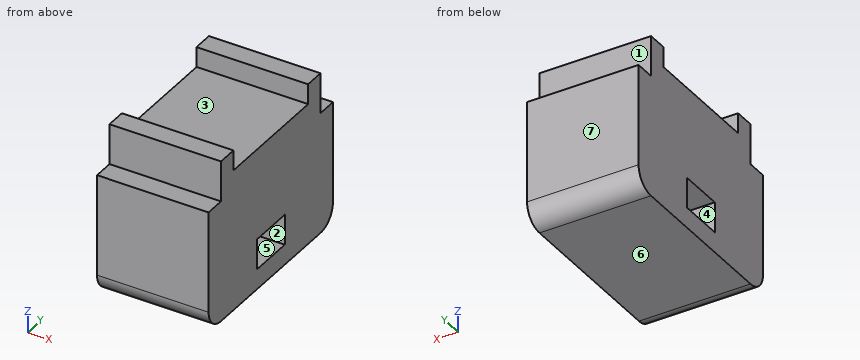
```python
from build123d import *

# Parameters (mm, degrees)
SKETCH1_W           = 20
SKETCH1_H           = 12
BOSS_EXTRUDE1_DEPTH = 11
SKETCH5_W           = 16
SKETCH5_H           = 11
BOSS_EXTRUDE2_DEPTH = 8
FILLET1_R           = 2
SKETCH7_W           = 4.5
SKETCH7_H           = 3
CUT_EXTRUDE1_DEPTH  = 15
SKETCH9_W           = 11
SKETCH9_H           = 2
BOSS_EXTRUDE4_DEPTH = 2


with BuildPart() as part:
    # Sketch1 → Boss-Extrude1 (new body)
    with BuildSketch(Plane.YZ):
        Rectangle(SKETCH1_W, SKETCH1_H)
    extrude(amount=BOSS_EXTRUDE1_DEPTH)

    # Sketch5 → Boss-Extrude2 (add)
    with BuildSketch(Plane(origin=(0, 0, 0), x_dir=(0, 1, 0), z_dir=(0, 0, 1))):
        with Locations((0, -5.5)):
            Rectangle(SKETCH5_W, SKETCH5_H)
    extrude(amount=BOSS_EXTRUDE2_DEPTH)

    # Fillet1
    fillet1_edges = [part.edges().sort_by_distance(p)[0] for p in [
        (5.5, 10, -6),
        (5.5, -10, -6),
    ]]
    fillet(fillet1_edges, radius=FILLET1_R)

    # Sketch7 → Cut-Extrude1 (cut)
    with BuildSketch(Plane.YZ):
        with Locations((0, -2.5)):
            Rectangle(SKETCH7_W, SKETCH7_H)
    extrude(amount=CUT_EXTRUDE1_DEPTH, mode=Mode.SUBTRACT)

    # Sketch9 → Boss-Extrude4 (add)
    with BuildSketch(Plane.XY.offset(8)):
        with Locations((5.5, 7)):
            Rectangle(SKETCH9_W, SKETCH9_H)
        with Locations((5.5, -7)):
            Rectangle(SKETCH9_W, SKETCH9_H)
    extrude(amount=BOSS_EXTRUDE4_DEPTH)


solid = part.part
```
CAD build for the part. Positions are in the model's coordinates, mm. Face numbers are marked on the shaded views. A direction names the side the tool comes from. Round coordinates to 2 decimals unless told otherwise and drop trailing zeros. Order: outer loops, then holes, each group sorted by start corner. A loop starts at its lowest first (then second) coordinate and runs counter-clockwise, first axis right, second up. Notation, with made-up numbers: (46, 30.5) - (51, 30.5) arc R14 ccw to (51, 38.5) - close; hole circle Ø10 at (43, 58.5). An arc over 180 degrees is marked (long way). Use CSV: the item, a comma, the result in double quotes. Start each with the question number.
1) Two-plate mould, pull along Z, no slides. Class the marked faces 4, 5, 6 and 7: pulls with the +Z half, pulls with the -Z half, needs draft (parallel to the pull), parting line crosses it, or undercut.
2) Saw through at B-B (y = 1). List the corners of the cut face in (x, z), and give its area (3 significant figures).
3) Saw through at D-D (y = 5.25). List the corners of the cut face in (x, z), and give its area (3 significant figures).
4) Saw through at A-A (z = -3.5). List the corners of the cut face in (x, y), and give its area (4 significant figures).
5) Pin check, flat tips, straight feed: pin 1 Ø1 at (y, z) = (7, 6.5) entering from -X; pin 2 Ø3.5 at (x, y) = (6.5, 0.5) entering from +Z; pin 3 Ø2 at (x, z) = (3, 8.5) entering from -Y; pin 4 Ø1.6 at (x, y) = (6.5, 9) entering from +Z. Stop position of each tip, or through.
6) Tool access for the marked faces 1, 2 and 3: list every direction of +Z, -Z, +X, -X, +Y, -Y with a clear straight run to the whole face (end or side of a thin tool).
7) Saw through at C-C (x = 4.25). List the corners of the cut face in (y, z).
8) Wall check: L1, parallel to Z at x = 4, y = 1.5; L2, parallel to Y at x = 5, z = -2; L3, parallel to Y at x = 8.25, z = 8.25. Give the ranges that are in metal, low to high. Write a range as [from, to].
Values follow:
1,face 4,"undercut"
1,face 5,"undercut"
1,face 6,"pulls with the -Z half"
1,face 7,"needs draft"
2,outline,"(0, -6) - (11, -6) - (11, -4) - (0, -4) - close; (0, -1) - (11, -1) - (11, 8) - (0, 8) - close"
2,area,"121 mm2"
3,outline,"(0, -6) - (11, -6) - (11, 8) - (0, 8) - close"
3,area,"154 mm2"
4,outline,"(0, -10) - (11, -10) - (11, -2.25) - (0, -2.25) - close; (0, 2.25) - (11, 2.25) - (11, 10) - (0, 10) - close"
4,area,"170.5 mm2"
5,pin 1,"stops at x = 0"
5,pin 2,"stops at z = 8"
5,pin 3,"stops at y = -8"
5,pin 4,"stops at z = 6"
6,face 1,"+Z, +X, -X, +Y"
6,face 2,"+X, -X"
6,face 3,"+Z, +X, -X"
7,outline,"(-10, -4) arc R2 ccw to (-8, -6) - (8, -6) arc R2 ccw to (10, -4) - (10, 6) - (8, 6) - (8, 10) - (6, 10) - (6, 8) - (-6, 8) - (-6, 10) - (-8, 10) - (-8, 6) - (-10, 6) - close; hole (-2.25, -4) - (2.25, -4) - (2.25, -1) - (-2.25, -1) - close"
8,L1,"z = [-6, -4], [-1, 8]"
8,L2,"y = [-10, -2.25], [2.25, 10]"
8,L3,"y = [-8, -6], [6, 8]"
